Can you work these out from the model? Positions are in its coordinate system, mm. A direction names the side the tool comes from. Give positions to 0.01 mm unless a question says otherwise; leave off trailing zeros. Order: outer loops, then holes, each group sorted by start corner. A loop starts at its lowest first (then second) coordinate and runs counter-clockwise, first axis right, second up. Notation, with made-up numbers: (28.25, 75) -> (53.25, 75) arc R23 ccw to (53.25, 112) -> close; hole circle Ø2 at (31.25, 45.25). An arc over 180 degrees is marked (long way). Answer as a JSON object with one key per item and string values.
```python
from build123d import *

# Parameters (mm, degrees)
BOSS_EXTRUDE1_DEPTH      = 5.08
BOSS_EXTRUDE1_DEPTH_BACK = 5.08
BOSS_EXTRUDE1_START      = -15.3035
FILLET1_R                = 12.7
FILLET2_R                = 12.7
FILLET3_R                = 25.4
BOSS_EXTRUDE2_DEPTH      = 10.16
CUT_EXTRUDE1_DEPTH       = 2.032
CUT_EXTRUDE1_DEPTH_BACK  = 2.032


with BuildPart() as part:
    # Sketch1 → Boss-Extrude1 (new, two sides: drawn at the far end of the back side and taken through both)
    with BuildSketch(Plane.XY.offset(132.610741806).offset(BOSS_EXTRUDE1_START - BOSS_EXTRUDE1_DEPTH_BACK)):
        Polygon((-83.578638746, 26.563044496), (-83.578638746, 12.034244496), (-71.412108995, 3.703044496), (-21.577168497, 3.703044496), (-9.410638746, 12.034244496), (-9.410638746, 26.563044496), (-9.410638746, 41.086800568), (-21.577168497, 59.456669294), (-71.412108995, 59.456669294), (-83.578638746, 41.086800568), align=None)
        Polygon((-65.266559293, 13.863044496), (-77.846462947, 22.47730801), (-77.846462947, 32.63730801), (-66.181452594, 49.296669294), (-26.807824897, 49.296669294), (-15.142814545, 32.63730801), (-15.142814545, 22.47730801), (-27.722718198, 13.863044496), align=None, mode=Mode.SUBTRACT)
    extrude(amount=BOSS_EXTRUDE1_DEPTH + BOSS_EXTRUDE1_DEPTH_BACK)

    # Fillet1
    fillet1_edges = [part.edges().sort_by_distance(p)[0] for p in [
        (-9.410638746, 41.086800568, 117.307241806),
    ]]
    fillet(fillet1_edges, radius=FILLET1_R)

    # Fillet2
    fillet2_edges = [part.edges().sort_by_distance(p)[0] for p in [
        (-83.578638746, 41.086800568, 117.307241806),
    ]]
    fillet(fillet2_edges, radius=FILLET2_R)

    # Fillet3
    fillet3_edges = [part.edges().sort_by_distance(p)[0] for p in [
        (-65.266559293, 13.863044496, 117.307241806),
        (-27.722718198, 13.863044496, 117.307241806),
        (-26.807824897, 49.296669294, 117.307241806),
        (-66.181452594, 49.296669294, 117.307241806),
    ]]
    fillet(fillet3_edges, radius=FILLET3_R)

    # Sketch2 → Boss-Extrude2 (add)
    with BuildSketch(Plane.XY.offset(122.387241806)):
        Polygon((-83.578638746, -3.617199432), (-71.412108995, 3.703044496), (-76.651458613, 7.290761818), (-83.578638746, 3.122880808), align=None)
    boss_extrude2 = extrude(amount=-BOSS_EXTRUDE2_DEPTH)

    # Mirror1: Boss-Extrude2 across plane
    add(boss_extrude2.mirror(Plane(origin=(-46.494638746, 0, 0), x_dir=(0, 0, 1), z_dir=(1, 0, 0))))

    # Sketch3 → Cut-Extrude1 (cut, two sides: drawn at the far end of the back side and taken through both)
    with BuildSketch(Plane(origin=(0, 0, 117.307241806), x_dir=(-1, 0, 0), z_dir=(0, 0, -1)).offset(-CUT_EXTRUDE1_DEPTH_BACK)):
        Polygon((24.891011245, 56.456669294), (68.21883105, 56.456669294), (79.016596447, 39.586472788), (68.21883105, 52.296669294), (24.891011245, 52.296669294), (14.093245849, 39.586472788), align=None)
        Polygon((79.016596447, 19.036634436), (79.016596447, 12.857149387), (70.121493391, 6.703044496), (22.988348904, 6.703044496), (14.093245849, 12.857149387), (14.093245849, 19.036634436), (26.029608579, 10.863044496), (67.080233717, 10.863044496), align=None)
    extrude(amount=CUT_EXTRUDE1_DEPTH + CUT_EXTRUDE1_DEPTH_BACK, mode=Mode.SUBTRACT)


solid = part.part
```
1. If we section it at C-C on y = 1: Please give me the cut outline in (x, z).
Worked answers:
{"outline": "(-83.58, 112.23) -> (-75.9, 112.23) -> (-75.9, 122.39) -> (-83.58, 122.39) -> close; (-17.08, 112.23) -> (-9.41, 112.23) -> (-9.41, 122.39) -> (-17.08, 122.39) -> close"}
2. If we section it at A-A on x = -31: Please give me the cut outline in (y, z), then the cut area to 3 significant figures.
Worked answers:
{"outline": "(3.7, 112.23) -> (14.28, 112.23) -> (14.28, 122.39) -> (3.7, 122.39) -> close; (47.64, 112.23) -> (59.46, 112.23) -> (59.46, 122.39) -> (47.64, 122.39) -> close; hole (6.7, 115.28) -> (10.86, 115.28) -> (10.86, 119.34) -> (6.7, 119.34) -> close; hole (52.3, 115.28) -> (56.46, 115.28) -> (56.46, 119.34) -> (52.3, 119.34) -> close", "area": "194 mm²"}
3. Will these pins go through, and if not, where does the flat tip stop? pin 1 Ø1.2 at (x, z) = (-46, 117.5) entering from -Y; pin 2 Ø6 at (x, z) = (-75.5, 117) entering from -Y.
Worked answers:
{"pin 1": "y = 3.7", "pin 2": "y = -0.56"}
4. For faces 1 (the face through (-12.92, 9.63, 117.24)), 2 (the face through (-77.58, -0.01, 117.38)), 3 (the face through (-47, 6.703, 117)), 4 (the face through (-80.164, 9.696, 117.236)), 5 (the face through (-15.143, 28, 117)), which set-ups out of +Z, -Z, +X, -X, +Y, -Y let a thin tool reach every point of the face, with its end or its side?
Worked answers:
{"face 1": "+Z, -Z, +X", "face 2": "+Z, -Z, -Y", "face 3": "none", "face 4": "+Z, -Z, -X", "face 5": "+Z, -Z"}
5. If we mould it in two halves opening along Y, with no side actions, what happens to faces 6 (the face through (-15.409, -0.008, 117.378)), 7 (the face through (-9.411, 0, 117)), 8 (the face through (-19.568, 46.031, 117.336))? For each: +Y half, -Y half, draft (parallel to the pull), parting line (faces both ways), or undercut.
Worked answers:
{"face 6": "-Y half", "face 7": "draft", "face 8": "undercut"}
6. If we section it at B-B on z = 121: Please give me the cut outline in (x, y), then the cut area to 3 significant figures.
Worked answers:
{"outline": "(-83.58, -3.62) -> (-71.41, 3.7) -> (-21.58, 3.7) -> (-9.41, -3.62) -> (-9.41, 3.12) -> (-16.34, 7.29) -> (-9.41, 12.03) -> (-9.41, 37.26) arc R12.7 ccw to (-11.52, 44.28) -> (-21.58, 59.46) -> (-71.41, 59.46) -> (-81.47, 44.28) arc R12.7 ccw to (-83.58, 37.26) -> (-83.58, 12.03) -> (-76.65, 7.29) -> (-83.58, 3.12) -> close; hole (-77.85, 22.48) -> (-71.75, 18.31) arc R25.4 ccw to (-57.4, 13.86) -> (-35.59, 13.86) arc R25.4 ccw to (-21.23, 18.31) -> (-15.14, 22.48) -> (-15.14, 32.64) -> (-19.22, 38.47) arc R25.4 ccw to (-40.03, 49.3) -> (-52.96, 49.3) arc R25.4 ccw to (-73.77, 38.47) -> (-77.85, 32.64) -> close", "area": "2,080 mm²"}
7. Please list where these lines run through material, in increasing order: L1, parallel to Y at x = -52.5, z = 115.5; L2, parallel to X at y = 23, z = 118.25; L3, parallel to Z at x = -44, y = 8.
Worked answers:
{"L1": "3.7 to 6.7, 10.86 to 13.86, 49.3 to 52.3, 56.46 to 59.46", "L2": "-83.58 to -77.85, -15.14 to -9.41", "L3": "112.23 to 115.28, 119.34 to 122.39"}
8. If we section it at D-D on y = 45.5: Please give me the cut outline in (x, z).
Worked answers:
{"outline": "(-80.66, 112.23) -> (-66.32, 112.23) -> (-66.32, 122.39) -> (-80.66, 122.39) -> close; (-26.67, 112.23) -> (-12.33, 112.23) -> (-12.33, 122.39) -> (-26.67, 122.39) -> close; hole (-75.23, 115.28) -> (-73.99, 115.28) -> (-73.99, 119.34) -> (-75.23, 119.34) -> close; hole (-19.12, 115.28) -> (-17.88, 115.28) -> (-17.88, 119.34) -> (-19.12, 119.34) -> close"}
